Design review of the part built by this model. Coordinates are the model's own, in mm. Face numbers are marked on the shaded views. A direction names the side the tool comes from. Round coordinates to 2 decimals unless told otherwise and drop trailing zeros. Order: outer loops, then holes, each group sorted by start corner. A loop starts at its lowest first (then second) coordinate and runs counter-clockwise, first axis right, second up. Notation, with made-up numbers: (-24.5, -30) - (9.5, -30) arc R26 cw to (9.5, 6) - close; hole circle Ø6 at (-20.75, -9.75). An arc over 180 degrees is marked (long way). Use CSV: the item, a comma, the result in double quotes.
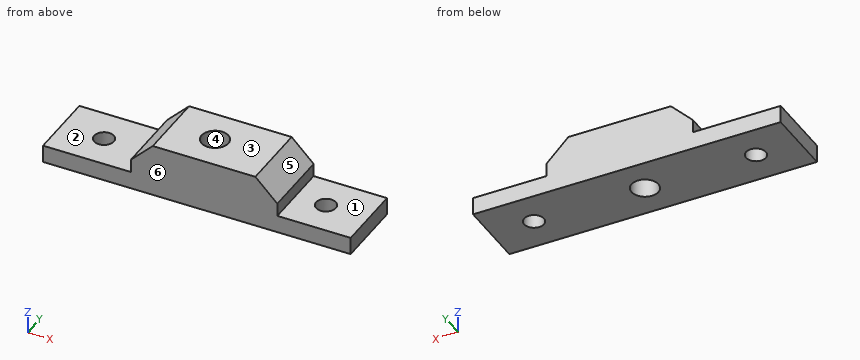
from build123d import *

# Parameters (mm, degrees)
F0_W     = 19.9736606702
F0_H     = 15.8
F0_R     = 2.25
F0_W_2   = 16.687778607
F0_W_3   = 33.3385607228
F0_R_2   = 3.05
F1_DEPTH = 4
F2_DEPTH = 12
F3_SIZE  = 5


with BuildPart() as f1:
    # F0 (on Top) → F1 (new body)
    with BuildSketch(Plane.XY):
        with Locations((-25.0131696649, -7.9)):
            Rectangle(F0_W, F0_H)
        with Locations((-25.25, -7.9)):
            Circle(F0_R, mode=Mode.SUBTRACT)
        with Locations((26.6561106965, -7.9)):
            Rectangle(F0_W_2, F0_H)
        with Locations((25.25, -7.9)):
            Circle(F0_R, mode=Mode.SUBTRACT)
        with Locations((1.6429410316, -7.9)):
            Rectangle(F0_W_3, F0_H)
        with Locations((0, -7.9)):
            Circle(F0_R_2, mode=Mode.SUBTRACT)
    extrude(amount=F1_DEPTH)

    # F0 (on Top) → F2 (join)
    with BuildSketch(Plane.XY):
        with Locations((1.6429410316, -7.9)):
            Rectangle(F0_W_3, F0_H)
        with Locations((0, -7.9)):
            Circle(F0_R_2, mode=Mode.SUBTRACT)
    extrude(amount=F2_DEPTH)

    # F3
    f3_edges = [f1.edges().sort_by_distance(p)[0] for p in [
        (-15.026339, -7.9, 12),
        (18.312221, -7.9, 12),
    ]]
    chamfer(f3_edges, length=F3_SIZE)


solid = f1.part
1) Insertion check: pin 1 Ø4 at (y, z) = (-13, 10.5) entering from +X; pin 2 Ø2.5 at (y, z) = (-12, 5.5) entering from +X; pin 3 Ø5.5 at (x, y) = (0, -7.9) entering from +Z; pin 4 Ø5 at (x, y) = (25.25, -7.9) entering from +Z. Each pin has a flat end and moves straight along its axis. Give the tip position at first contact, or say it passes through.
Data:
pin 1,"stops at x = 16.81"
pin 2,"stops at x = 18.31"
pin 3,"passes through"
pin 4,"stops at z = 4"
2) For the marked faces 1, 2 and 3, list the 3-axis set-ups (+Z, -Z, +X, -X, +Y, -Y) from which the entire face can be reached by the end or side of a thin tool; tool diameter is ignored.
Data:
face 1,"+Z, +X, +Y, -Y"
face 2,"+Z, -X, +Y, -Y"
face 3,"+Z, +X, -X, +Y, -Y"
3) We need section D-D (y = -12.5). Give the boundary of the cut face in (x, z).
Data:
outline,"(-35, 0) - (35, 0) - (35, 4) - (18.31, 4) - (18.31, 7) - (13.31, 12) - (-10.03, 12) - (-15.03, 7) - (-15.03, 4) - (-35, 4) - close"
4) To check wall thickness, follow L1, parallel to Y at x = 0, z = 9.75; L2, parallel to Y at x = -25.25, z = 1.6; L3, parallel to Z at x = -21.5, y = -14. State the ranges of each line that lie inside material, in increasing order. Write a range as from..to.
Data:
L1,"y = -15.8..-10.95, -4.85..0"
L2,"y = -15.8..-10.15, -5.65..0"
L3,"z = 0..4"
5) The part is to be moulded in two halves that separate along X. For the marked faces 4, 5 and 6, say which applies: +X half, -X half, draft (parallel to the pull), parting line (faces both ways), or undercut.
Data:
face 4,"undercut"
face 5,"+X half"
face 6,"draft"
6) We need section A-A (y = -7.9). Give the boundary of the cut face in (x, z).
Data:
outline,"(-35, 0) - (-27.5, 0) - (-27.5, 4) - (-35, 4) - close; (-23, 0) - (-3.05, 0) - (-3.05, 12) - (-10.03, 12) - (-15.03, 7) - (-15.03, 4) - (-23, 4) - close; (3.05, 0) - (23, 0) - (23, 4) - (18.31, 4) - (18.31, 7) - (13.31, 12) - (3.05, 12) - close; (27.5, 0) - (35, 0) - (35, 4) - (27.5, 4) - close"
7) We need section B-B (x = 0). Give the boundary of the cut face in (y, z).
Data:
outline,"(-15.8, 0) - (-10.95, 0) - (-10.95, 12) - (-15.8, 12) - close; (-4.85, 0) - (0, 0) - (0, 12) - (-4.85, 12) - close"
8) We need section C-C (z = 1). Give the boundary of the cut face in (x, y), then the cut area to 3 significant figures.
Data:
outline,"(-35, -15.8) - (35, -15.8) - (35, 0) - (-35, 0) - close; hole circle Ø4.5 at (-25.25, -7.9); hole circle Ø6.1 at (0, -7.9); hole circle Ø4.5 at (25.25, -7.9)"
area,"1,040 mm2"
